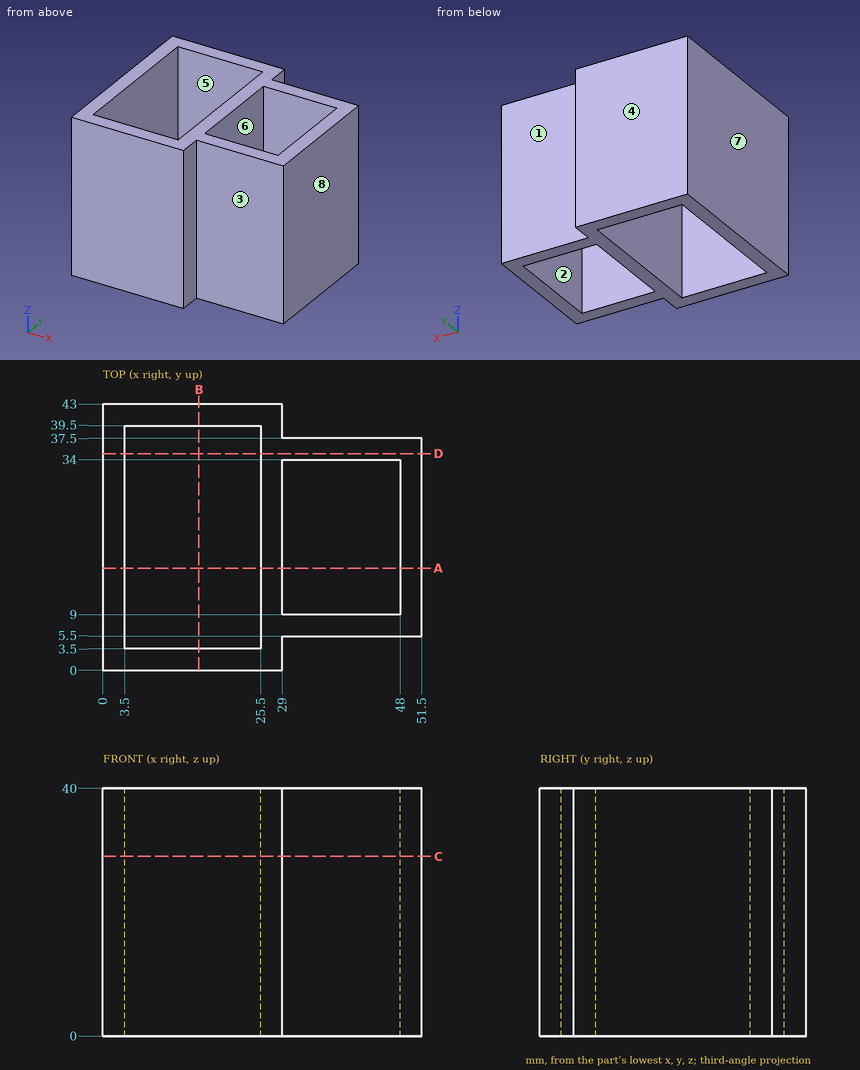
Input: dimensioned drawing with shaded views. Units: mm. Origin: part minimum x, y, z. A direction names the side the tool comes from. Round coordinates to 2 decimals unless told otherwise and drop trailing zeros. Order: outer loops, then holes, each group sorted by start corner. A loop starts at its lowest first (then second) coordinate and runs counter-clockwise, first axis right, second up. Notation, with made-up numbers: (-31, 42.5) -> (13, 42.5) arc R35 ccw to (13, 79.5) -> close; hole circle Ø3 at (-38.75, 16.5). An arc over 180 degrees is marked (long way). One line per item, written item: value. Start each with the question number.
Q1. Pin query (flat end, axial travel): pin 1 (4.5 mm diameter, centred on y = 41, z = 13, fed in from +X); pin 2 (4 mm diameter, centred on x = 40.5, z = 26.5, fed in from -Y); pin 3 (1 mm diameter, centred on x = 30, z = 9, fed in from +Y); pin 4 (2 mm diameter, centred on x = 23.5, y = 8, fed in from +Z). Return the tip coordinate at first contact, or that it passes through.
Q2. Section query A-A (y = 16.5). Return the cut outline in (x, z), plus the area to 3 significant figures.
Q3. Section query B-B (x = 15.5). Return the cut outline in (y, z).
Q4. Draft query along X for the marked faces 5, 6, 7 and 8. Return one class per face: pulls with the +X half, pulls with the -X half, needs draft (parallel to the pull), parting line crosses it, or undercut.
Q5. Section query C-C (z = 29). Return the cut outline in (x, y), plus the area to 3 significant figures.
Q6. Access query for the marked faces 1, 2, 3 and 4. Directions: +Z, -Z, +X, -X, +Y, -Y. A direction counts if a zero-diameter tool reaches every point of the face in a straight line with its end or side. Return the directions, or none.
Q7. Material intervals for probe 1 along X at (y, z) = (14, 6); probe 2 along X at (y, z) = (8.5, 27.5); probe 3 along Y at (x, z) = (5, 25.5), sorted ascending.
Q8. Section query D-D (y = 35). Return the cut outline in (x, z), plus the area to 3 significant figures.
Findings below:
1. pin 1: x = 29
1. pin 2: y = 5.5
1. pin 3: y = 37.5
1. pin 4: through
2. outline: (0, 0) -> (3.5, 0) -> (3.5, 40) -> (0, 40) -> close; (25.5, 0) -> (29, 0) -> (29, 40) -> (25.5, 40) -> close; (48, 0) -> (51.5, 0) -> (51.5, 40) -> (48, 40) -> close
2. area: 420 mm²
3. outline: (0, 0) -> (3.5, 0) -> (3.5, 40) -> (0, 40) -> close; (39.5, 0) -> (43, 0) -> (43, 40) -> (39.5, 40) -> close
4. face 5: undercut
4. face 6: undercut
4. face 7: pulls with the -X half
4. face 8: pulls with the +X half
5. outline: (0, 0) -> (29, 0) -> (29, 5.5) -> (51.5, 5.5) -> (51.5, 37.5) -> (29, 37.5) -> (29, 43) -> (0, 43) -> close; hole (3.5, 3.5) -> (25.5, 3.5) -> (25.5, 39.5) -> (3.5, 39.5) -> close; hole (29, 9) -> (48, 9) -> (48, 34) -> (29, 34) -> close
5. area: 700 mm²
6. face 1: +Z, -Z, +X, +Y
6. face 2: +Z, -Z
6. face 3: +Z, -Z, +X, -Y
6. face 4: +Z, -Z, +X, -X, +Y
7. probe 1: 0 to 3.5, 25.5 to 29, 48 to 51.5
7. probe 2: 0 to 3.5, 25.5 to 51.5
7. probe 3: 0 to 3.5, 39.5 to 43
8. outline: (0, 0) -> (3.5, 0) -> (3.5, 40) -> (0, 40) -> close; (25.5, 0) -> (51.5, 0) -> (51.5, 40) -> (25.5, 40) -> close
8. area: 1,180 mm²
